from build123d import *

# Parameters (mm, degrees)
SKETCH1_W                            = 159.7
SKETCH1_H                            = 109.7
SKETCH1_W_2                          = 144.2
SKETCH1_H_2                          = 103.2
BOSS_EXTRUDE1_DEPTH                  = 11
F_2_4_2_4_DIAMETER_HOLE1_D           = 2.4
CUT_EXTRUDE10_DEPTH                  = 3.5
LPATTERN1_COUNT                      = 2
LPATTERN1_PITCH                      = 72
MIRROR2_COPY_1_DEPTH                 = 3.5
M2X0_4_TAPPED_HOLE1_D                = 1.6
M2X0_4_TAPPED_HOLE1_DEPTH            = 3.5
M2X0_4_TAPPED_HOLE1_CSINK_D          = 2.05
M2X0_4_TAPPED_HOLE1_CSINK_ANGLE      = 90
M2X0_4_TAPPED_HOLE1_TIP              = 0.480688495
SKETCH11_W                           = 4.35
SKETCH11_H                           = 6
CUT_EXTRUDE4_DEPTH                   = 3.5
CUT_EXTRUDE11_DEPTH                  = 98.16375353
CUT_EXTRUDE11_DEPTH_BACK             = 98.16375353
F_2_4_2_4_DIAMETER_HOLE2_D           = 2.4
F_2_7_2_7_DIAMETER_HOLE1_D           = 2.7
F_2_7_2_7_DIAMETER_HOLE1_CSINK_D     = 2.75
F_2_7_2_7_DIAMETER_HOLE1_CSINK_ANGLE = 90
CUT_EXTRUDE6_DEPTH                   = 98.496384548
SKETCH19_R                           = 1.6
CUT_EXTRUDE7_DEPTH                   = 3.5
CUT_EXTRUDE8_DEPTH                   = 98.496384548
SKETCH8_R                            = 8
CUT_EXTRUDE9_DEPTH                   = 98.496384548
FILLET1_R                            = 2
FILLET2_R                            = 8
FILLET3_R                            = 1
FILLET4_R                            = 2
FILLET5_R                            = 0.5
CUT_EXTRUDE13_REACH                  = 138.129
SKETCH33_W                           = 130
SKETCH33_H                           = 6.2
SKETCH34_W                           = 4.2
SKETCH34_H                           = 4.2
CUT_EXTRUDE14_DEPTH                  = 2.5
MIRROR5_COPY_1_SKETCH_W              = 4.2
MIRROR5_COPY_1_SKETCH_H              = 4.2
MIRROR5_COPY_1_DEPTH                 = 2.5
SKETCH35_R                           = 1.75
CUT_EXTRUDE15_DEPTH                  = 4.5
SKETCH38_R                           = 1.25
CUT_EXTRUDE17_DEPTH                  = 98.091683475


with BuildPart() as part:
    # Sketch1 → Boss-Extrude1 (new body)
    with BuildSketch(Plane(origin=(0, 0, 0), x_dir=(1, 0, 0), z_dir=(0, 1, 0))):
        Rectangle(SKETCH1_W, SKETCH1_H)
        Rectangle(SKETCH1_W_2, SKETCH1_H_2, mode=Mode.SUBTRACT)
    extrude(amount=BOSS_EXTRUDE1_DEPTH)

    # Ø2.4 (2.4) Diameter Hole1 (through all)
    with Locations(Plane(origin=(0, 11, 0), x_dir=(1, 0, 0), z_dir=(0, 1, 0))):
        with Locations((-77.5, 36), (77.5, 36), (-77.5, -36), (77.5, -36)):
            Hole(F_2_4_2_4_DIAMETER_HOLE1_D / 2)

    # Sketch29 → Cut-Extrude10 (cut)
    with BuildSketch(Plane(origin=(0, 11, 0), x_dir=(1, 0, 0), z_dir=(0, 1, 0))):
        with BuildLine():
            Line((-77.5, 38), (-79.85, 38))
            Line((-79.85, 38), (-79.85, 34))
            Line((-79.85, 34), (-77.5, 34))
            ThreePointArc((-77.5, 34), (-75.5, 36), (-77.5, 38))
        make_face()
    cut_extrude10 = extrude(amount=-CUT_EXTRUDE10_DEPTH, mode=Mode.SUBTRACT)

    # LPattern1: Cut-Extrude10 ×2
    with Locations(*[(0, 0, i * LPATTERN1_PITCH) for i in range(1, LPATTERN1_COUNT)]):
        add(cut_extrude10, mode=Mode.SUBTRACT)

    # Mirror2: Cut-Extrude10 across plane
    add(cut_extrude10.mirror(Plane(origin=(0, 0, 0), x_dir=(0, 0, 1), z_dir=(1, 0, 0))), mode=Mode.SUBTRACT)

    # Mirror2 copy 1 sketch → Mirror2 copy 1 (cut)
    with BuildSketch(Plane(origin=(0, 11, 72), x_dir=(-1, 0, 0), z_dir=(0, 1, 0))):
        with BuildLine():
            Line((-77.5, -38), (-79.85, -38))
            Line((-79.85, -38), (-79.85, -34))
            Line((-79.85, -34), (-77.5, -34))
            ThreePointArc((-77.5, -34), (-75.5, -36), (-77.5, -38))
        make_face()
    extrude(amount=-MIRROR2_COPY_1_DEPTH, mode=Mode.SUBTRACT)

    # M2x0.4 Tapped Hole1
    with Locations(Plane(origin=(0, 11, 0), x_dir=(1, 0, 0), z_dir=(0, 1, 0))):
        with Locations((-74, 40), (-74, -40), (74, 40), (74, -40)):
            CounterSinkHole(M2X0_4_TAPPED_HOLE1_D / 2, M2X0_4_TAPPED_HOLE1_CSINK_D / 2, depth=M2X0_4_TAPPED_HOLE1_DEPTH, counter_sink_angle=M2X0_4_TAPPED_HOLE1_CSINK_ANGLE)
            with Locations((0, 0, -(M2X0_4_TAPPED_HOLE1_DEPTH + M2X0_4_TAPPED_HOLE1_TIP / 2))):  # 118° drill point
                Cone(0, M2X0_4_TAPPED_HOLE1_D / 2, M2X0_4_TAPPED_HOLE1_TIP, mode=Mode.SUBTRACT)

    # Sketch11 → Cut-Extrude4 (cut)
    with BuildSketch(Plane(origin=(0, 11, 0), x_dir=(1, 0, 0), z_dir=(0, 1, 0))):
        with Locations((-77.675, 39)):
            Rectangle(SKETCH11_W, SKETCH11_H)
    extrude(amount=-CUT_EXTRUDE4_DEPTH, mode=Mode.SUBTRACT)

    # Sketch30 → Cut-Extrude11 (cut, two sides: drawn at the far end of the back side and taken through both)
    with BuildSketch(Plane(origin=(0, 7.5, 0), x_dir=(1, 0, 0), z_dir=(0, 1, 0)).offset(-CUT_EXTRUDE11_DEPTH_BACK)):
        with BuildLine():
            Line((-75.5, 40), (-75.5, 42))
            Line((-75.5, 42), (-79.85, 42))
            Line((-79.85, 42), (-79.85, 38))
            Line((-79.85, 38), (-77.5, 38))
            ThreePointArc((-77.5, 38), (-76.085786438, 38.585786438), (-75.5, 40))
        make_face()
    extrude(amount=CUT_EXTRUDE11_DEPTH + CUT_EXTRUDE11_DEPTH_BACK, mode=Mode.SUBTRACT)

    # Ø2.4 (2.4) Diameter Hole2 (through all)
    with Locations(Plane(origin=(0, 11, 0), x_dir=(1, 0, 0), z_dir=(0, 1, 0))):
        with Locations((-77.5, -40), (77.5, 40), (77.5, -40)):
            Hole(F_2_4_2_4_DIAMETER_HOLE2_D / 2)

    # Ø2.7 (2.7) Diameter Hole1 (through all)
    with Locations(Plane(origin=(0, 11, 0), x_dir=(1, 0, 0), z_dir=(0, 1, 0))):
        with Locations((-77.5, 29), (-77.5, -29), (77.5, 29), (77.5, -29)):
            CounterSinkHole(F_2_7_2_7_DIAMETER_HOLE1_D / 2, F_2_7_2_7_DIAMETER_HOLE1_CSINK_D / 2, counter_sink_angle=F_2_7_2_7_DIAMETER_HOLE1_CSINK_ANGLE)

    # Sketch18 → Cut-Extrude6 (cut, through all)
    with BuildSketch(Plane(origin=(0, 11, 0), x_dir=(1, 0, 0), z_dir=(0, 1, 0))):
        with BuildLine():
            Line((-78.85, 24.85), (-79.85, 24.85))
            Line((-79.85, 24.85), (-79.85, 18.85))
            Line((-79.85, 18.85), (-78.85, 18.85))
            ThreePointArc((-78.85, 18.85), (-77.435786438, 19.435786438), (-76.85, 20.85))
            Line((-76.85, 20.85), (-76.85, 22.85))
            ThreePointArc((-76.85, 22.85), (-77.435786438, 24.264213562), (-78.85, 24.85))
        make_face()
    extrude(amount=-CUT_EXTRUDE6_DEPTH, mode=Mode.SUBTRACT)

    # Sketch19 → Cut-Extrude7 (cut)
    with BuildSketch(Plane(origin=(0, 11, 0), x_dir=(1, 0, 0), z_dir=(0, 1, 0))):
        with Locations(Location((77.35, 44.85, 0), (0, 0, 270))):
            Circle(SKETCH19_R)
        with Locations(Location((-77.35, -44.85, 0), (0, 0, 270))):
            Circle(SKETCH19_R)
    extrude(amount=-CUT_EXTRUDE7_DEPTH, mode=Mode.SUBTRACT)

    # Sketch7 → Cut-Extrude8 (cut, through all)
    with BuildSketch(Plane(origin=(0, 11, 0), x_dir=(1, 0, 0), z_dir=(0, 1, 0))):
        with BuildLine():
            Line((-76.85, 48.85), (-79.85, 48.85))
            Line((-79.85, 48.85), (-79.85, 40.85))
            Line((-79.85, 40.85), (-76.85, 40.85))
            ThreePointArc((-76.85, 40.85), (-72.85, 44.85), (-76.85, 48.85))
        make_face()
    extrude(amount=-CUT_EXTRUDE8_DEPTH, mode=Mode.SUBTRACT)

    # Sketch8 → Cut-Extrude9 (cut, through all)
    with BuildSketch(Plane(origin=(0, 11, 0), x_dir=(1, 0, 0), z_dir=(0, 1, 0))):
        with Locations((-79.85, -54.85)):
            Circle(SKETCH8_R)
    extrude(amount=-CUT_EXTRUDE9_DEPTH, mode=Mode.SUBTRACT)

    # Fillet1
    fillet1_edges = [part.edges().sort_by_distance(p)[0] for p in [
        (72.1, 5.5, 51.6),
        (72.1, 5.5, -51.6),
        (-72.1, 5.5, -51.6),
        (-72.1, 5.5, 51.6),
    ]]
    fillet(fillet1_edges, radius=FILLET1_R)

    # Fillet2
    # the kernel refuses this fillet: 8 mm, written as the material it takes off along each edge
    with BuildSketch(Plane(origin=(79.85, -20, 54.85), x_dir=(-1, 0, 0), z_dir=(0, 1, 0)), Plane(origin=(79.85, -20, -54.85), x_dir=(0, 0, 1), z_dir=(0, 1, 0))) as fillet2_piece_1:
        with BuildLine():
            CenterArc((FILLET2_R, -FILLET2_R), FILLET2_R, 90, 90)
            Line((0, -FILLET2_R), (-FILLET2_R * 0.02, -FILLET2_R))
            Line((-FILLET2_R * 0.02, -FILLET2_R), (-FILLET2_R * 0.02, FILLET2_R * 0.02))
            Line((-FILLET2_R * 0.02, FILLET2_R * 0.02), (FILLET2_R, FILLET2_R * 0.02))
            Line((FILLET2_R, FILLET2_R * 0.02), (FILLET2_R, 0))
        make_face()
    extrude(amount=51, mode=Mode.SUBTRACT)
    with BuildSketch(Plane(origin=(-79.85, -19.364916731, -54.85), x_dir=(1, 0, 0), z_dir=(0, 1, 0))) as fillet2_piece_2:
        with BuildLine():
            CenterArc((7.745966692, -8), FILLET2_R, 90, 75.522487814)
            Line((0, -6), (-0.154919334, -5.96))
            ThreePointArc((-0.154919334, -5.96), (-0.16, -3), (-0.16, 0))
            Line((-0.16, 0), (0, 0.16))
            Line((0, 0.16), (7.745966692, 0.16))
            Line((7.745966692, 0.16), (7.745966692, 0))
        make_face()
    extrude(amount=49.729833462, mode=Mode.SUBTRACT)

    # Fillet3
    fillet3_edges = [part.edges().sort_by_distance(p)[0] for p in [
        (-79.85, 5.5, -48.85),
        (-71.85, 5.5, 54.85),
        (-79.85, 5.5, 46.85),
    ]]
    fillet(fillet3_edges, radius=FILLET3_R)

    # Fillet4
    fillet4_edges = [part.edges().sort_by_distance(p)[0] for p in [
        (-79.85, 3.75, -38),
    ]]
    fillet(fillet4_edges, radius=FILLET4_R)

    # Fillet5
    fillet5_edges = [part.edges().sort_by_distance(p)[0] for p in [
        (-79.85, 5.5, -18.85),
        (-79.85, 5.5, -24.85),
    ]]
    fillet(fillet5_edges, radius=FILLET5_R)

    # Sketch33 → Cut-Extrude13 (cut, up to next)
    with BuildSketch(Plane.XY.offset(54.85), mode=Mode.PRIVATE) as cut_extrude13_sk1:
        with Locations((0.472135955, 7.9)):
            Rectangle(SKETCH33_W, SKETCH33_H)
    cut_extrude13_tool1 = extrude(cut_extrude13_sk1.sketch, amount=-CUT_EXTRUDE13_REACH, mode=Mode.PRIVATE) & part.part
    add(cut_extrude13_tool1.solids().sort_by_distance((0.472136, 7.9, 54.85))[0], mode=Mode.SUBTRACT)

    # Sketch34 → Cut-Extrude14 (cut)
    with BuildSketch(Plane(origin=(0, 0, 0), x_dir=(-1, 0, 0), z_dir=(0, -1, 0))):
        with Locations((-77.5, -29)):
            Rectangle(SKETCH34_W, SKETCH34_H)
    cut_extrude14 = extrude(amount=-CUT_EXTRUDE14_DEPTH, mode=Mode.SUBTRACT)

    # Mirror4: Cut-Extrude14 across plane
    add(cut_extrude14.mirror(Plane.XY), mode=Mode.SUBTRACT)

    # Mirror5: Cut-Extrude14 across plane
    add(cut_extrude14.mirror(Plane(origin=(0, 0, 0), x_dir=(0, 0, 1), z_dir=(1, 0, 0))), mode=Mode.SUBTRACT)

    # Mirror5 copy 1 sketch → Mirror5 copy 1 (cut)
    with BuildSketch(Plane.XZ):
        with Locations((-77.5, -29)):
            Rectangle(MIRROR5_COPY_1_SKETCH_W, MIRROR5_COPY_1_SKETCH_H)
    extrude(amount=-MIRROR5_COPY_1_DEPTH, mode=Mode.SUBTRACT)

    # Sketch35 → Cut-Extrude15 (cut)
    with BuildSketch(Plane(origin=(0, 11, 0), x_dir=(1, 0, 0), z_dir=(0, 1, 0))):
        with Locations(Location((-76.85, 0, 0), (0, 0, 270))):
            Circle(SKETCH35_R)
    cut_extrude15 = extrude(amount=-CUT_EXTRUDE15_DEPTH, mode=Mode.SUBTRACT)

    # Sketch38 → Cut-Extrude17 (cut, through all)
    with BuildSketch(Plane(origin=(0, 6.5, 0), x_dir=(1, 0, 0), z_dir=(0, 1, 0))):
        with Locations(Location((-76.85, 0, 0), (0, 0, 270))):
            Circle(SKETCH38_R)
    cut_extrude17 = extrude(amount=-CUT_EXTRUDE17_DEPTH, mode=Mode.SUBTRACT)

    # Mirror7: Cut-Extrude15, Cut-Extrude17 across plane
    add(cut_extrude15.mirror(Plane(origin=(0, 0, 0), x_dir=(0, 0, 1), z_dir=(1, 0, 0))), mode=Mode.SUBTRACT)
    add(cut_extrude17.mirror(Plane(origin=(0, 0, 0), x_dir=(0, 0, 1), z_dir=(1, 0, 0))), mode=Mode.SUBTRACT)


solid = part.part
Work out the finished part from the listing and answer in its coordinate system (mm). A direction names the side the tool comes from. Give positions to 0.01 mm unless a question says otherwise; leave off trailing zeros. Order: outer loops, then holes, each group sorted by start corner. A loop starts at its lowest first (then second) coordinate and runs counter-clockwise, first axis right, second up. Notation, with made-up numbers: (-20, 72.5) - (38, 72.5) arc R19 cw to (38, 77.5) - close; hole circle Ø4 at (-28.75, 59.5). An arc over 180 degrees is marked (long way). Answer as CSV lines item,"result". Start each with the question number.
Q1. Given pin 1 Ø2.5 at (x, z) = (77, -45.5) entering from +Y; pin 2 Ø4 at (x, y) = (-6.5, 9.5) entering from +Z; pin 3 Ø1.9 at (x, y) = (78.5, 9.5) entering from +Z; pin 4 Ø0.8 at (x, y) = (-77.5, 5) entering from +Z, each flat-ended and moving along its own axis, determine where each tip first touches the part or whether it passes through.
Q2. The part is cut by section A-A (z = 17). Write down the section's boundary in (x, y).
Q3. Find the intervals of material crossed by L1, parallel to X at y = 9.65, z = 44.85; L2, parallel to X at y = 7.25, z = -29; L3, parallel to X at y = 9.15, z = 40, in increasing order. Write a range as [from, to].
Q4. For faces 1 (the face through (79, 2.5, -29)), 2 (the face through (-75.115, 8.782, -0.228)), 3 (the face through (-72.1, 5, 1)), determine the directions among +Z, -Z, +X, -X, +Y, -Y from which every point of the face is accessible in a straight line to the end or side of a thin tool.
Q5. The part is cut by section B-B (x = -9). Write down the section's boundary in (y, z).
Q6. The mould has two halves that part along X. Classify faces 4 (the face through (-1, 2, 54.85)), 5 (the face through (-77, 7.5, 45)), 6 (the face through (-75.5, 9.3, 36)): +X half, -X half, draft (parallel to the pull), parting line (faces both ways), or undercut.
Check result:
1,pin 1,"stops at y = 11"
1,pin 2,"stops at z = -51.6"
1,pin 3,"stops at z = 52.46"
1,pin 4,"stops at z = 47.34"
2,outline,"(-79.85, 0) - (-72.1, 0) - (-72.1, 11) - (-79.85, 11) - close; (72.1, 0) - (79.85, 0) - (79.85, 11) - (72.1, 11) - close"
3,L1,"x = [-79.85, -78.95], [-75.75, -72.1], [72.1, 79.85]"
3,L2,"x = [-79.85, -78.85], [-76.15, -72.1], [72.1, 76.15], [78.85, 79.85]"
3,L3,"x = [-79.85, -78.7], [-76.3, -74.8], [-73.2, -72.1], [72.1, 73.2], [74.8, 76.3], [78.7, 79.85]"
4,face 1,"-Y"
4,face 2,"+Y"
4,face 3,"+Y, -Y"
5,outline,"(0, -54.85) - (11, -54.85) - (11, -51.6) - (0, -51.6) - close; (0, 51.6) - (4.8, 51.6) - (4.8, 54.85) - (0, 54.85) - close"
6,face 4,"draft"
6,face 5,"undercut"
6,face 6,"-X half"
